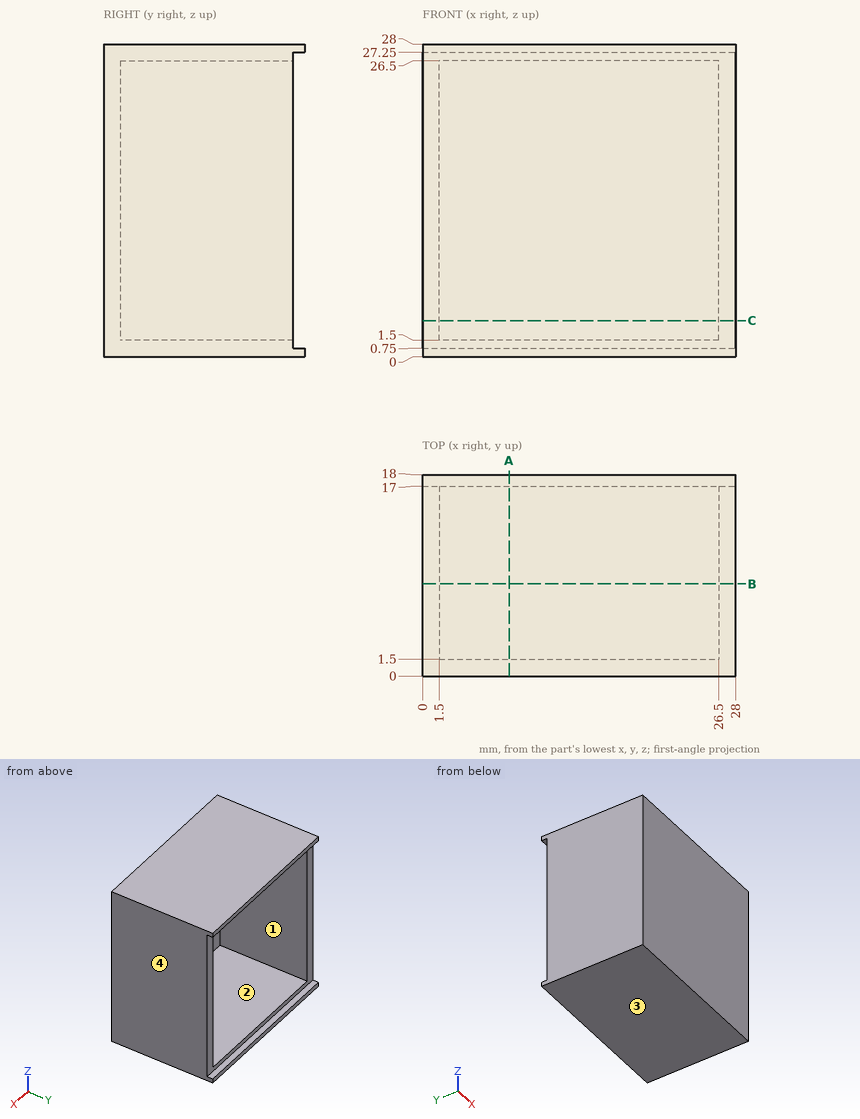
Can you work these out from the drawing? Everything is in mm from the part's minimum corner. Round coordinates to 2 decimals unless told otherwise and drop trailing zeros. Loops run counter-clockwise (first coordinate to the right, second up) from the corner with the lowest first, then second, coordinate; pieces in that order, holes last. Notation, with made-up numbers: (31, -25) -> (88, -25) arc R33 ccw to (88, 8) -> close; hole circle Ø2 at (55.25, 65.5). An arc over 180 degrees is marked (long way). Use CSV: the item, a comma, the result in double quotes.
(1) If we mould it in two halves opening along Z, with no side actions, what happens to the marked faces 1, 2, 3 and 4? For each: +Z half, -Z half, draft (parallel to the pull), parting line (faces both ways), or undercut.
Return value:
face 1,"undercut"
face 2,"undercut"
face 3,"-Z half"
face 4,"draft"
(2) Suppose I cut it at A-A on x = 7.75. Write out the boundary of the cut face in (y, z).
Return value:
outline,"(0, 0) -> (18, 0) -> (18, 0.75) -> (17, 0.75) -> (17, 1.5) -> (1.5, 1.5) -> (1.5, 26.5) -> (17, 26.5) -> (17, 27.25) -> (18, 27.25) -> (18, 28) -> (0, 28) -> close"
(3) Suppose I cut it at C-C on z = 3.25. Write out the boundary of the cut face in (x, y), plus the area to 3 significant figures.
Return value:
outline,"(0, 0) -> (28, 0) -> (28, 17) -> (26.5, 17) -> (26.5, 1.5) -> (1.5, 1.5) -> (1.5, 17) -> (0, 17) -> close"
area,"88.5 mm²"
(4) Suppose I cut it at B-B on y = 8.25. Write out the boundary of the cut face in (x, z), plus the area to 3 significant figures.
Return value:
outline,"(0, 0) -> (28, 0) -> (28, 28) -> (0, 28) -> close; hole (1.5, 1.5) -> (26.5, 1.5) -> (26.5, 26.5) -> (1.5, 26.5) -> close"
area,"159 mm²"
(5) Will these pins go through, and if not, where does the flat tip stop? pin 1 Ø1.5 at (x, z) = (17.5, 4) entering from +Y; pin 2 Ø5 at (x, y) = (14.5, 9.5) entering from -Z.
Return value:
pin 1,"stops at y = 1.5"
pin 2,"stops at z = 0"
(6) If I drill on probe 1 along X at (y, z) = (3.75, 12.75); probe 2 along Y at (x, z) = (26, 24.5), over which ranges is the centre line in solid material (lowest first)? Write a range as [from, to].
Return value:
probe 1,"x = [0, 1.5], [26.5, 28]"
probe 2,"y = [0, 1.5]"
